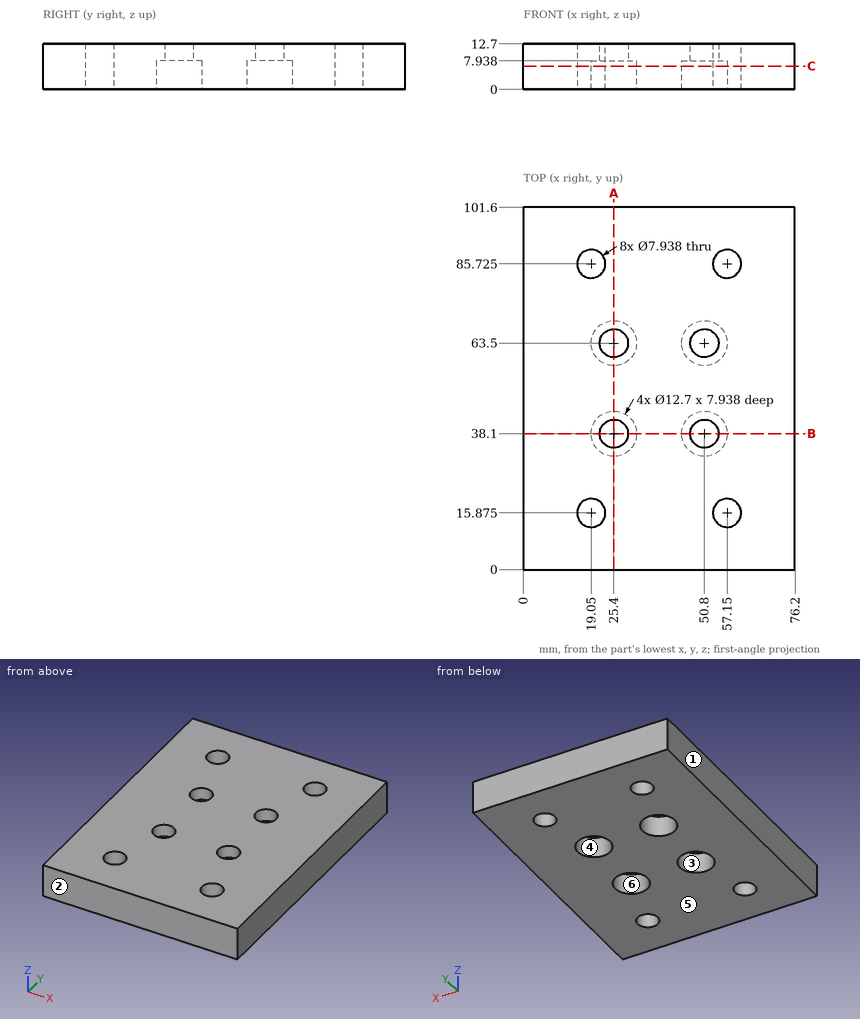
Part print with two shaded views. Sizes in mm from the minimum x, y, z corner. A direction names the side the tool comes from. Give positions to 0.01 mm unless a question says otherwise; leave off trailing zeros. Order: outer loops, then holes, each group sorted by start corner. A loop starts at its lowest first (then second) coordinate and runs counter-clockwise, first axis right, second up. Notation, with made-up numbers: M -37,-27.75 L -25,-27.75 A25 cw -25,-6.75 Z; hole C 8,9.5 d3. An arc over 180 degrees is marked long. Put each result on its own line as item: value.
Item 1: Drop a flat-ended pin along its axis: pin 1 Ø12.5 at (x, y) = (50.8, 63.5) entering from -Z. Give the stop position or say it passes through.
Results are:
pin 1: z = 7.94
Item 2: Cut at A-A on x = 25.4. Write the cut outline in (y, z).
Results are:
outline: M 0,0 L 31.75,0 L 31.75,7.94 L 34.13,7.94 L 34.13,12.7 L 0,12.7 Z; M 42.07,7.94 L 44.45,7.94 L 44.45,0 L 57.15,0 L 57.15,7.94 L 59.53,7.94 L 59.53,12.7 L 42.07,12.7 Z; M 67.47,7.94 L 69.85,7.94 L 69.85,0 L 101.6,0 L 101.6,12.7 L 67.47,12.7 Z
Item 3: Wall check: probe 1 along Y at (x, z) = (50.8, 9.3); probe 2 along X at (y, z) = (83, 2.5) (1 decimal); probe 3 along Y at (x, z) = (58.5, 5). Give the ranges that are in metal, low to high.
Results are:
probe 1: 0 to 34.13, 42.07 to 59.53, 67.47 to 101.6
probe 2: 0 to 16.2, 21.9 to 54.3, 60 to 76.2
probe 3: 0 to 12.14, 19.61 to 81.99, 89.46 to 101.6
Item 4: Cut at B-B on y = 38.1. Write the cut outline in (x, z).
Results are:
outline: M 0,0 L 19.05,0 L 19.05,7.94 L 21.43,7.94 L 21.43,12.7 L 0,12.7 Z; M 29.37,7.94 L 31.75,7.94 L 31.75,0 L 44.45,0 L 44.45,7.94 L 46.83,7.94 L 46.83,12.7 L 29.37,12.7 Z; M 54.77,7.94 L 57.15,7.94 L 57.15,0 L 76.2,0 L 76.2,12.7 L 54.77,12.7 Z
Item 5: Pull direction Y, two halves, no side cores. Call the marked faces 1, 2, 3 and 4: +Y half, -Y half, draft (parallel to the pull), parting line (faces both ways), or undercut.
Results are:
face 1: draft
face 2: -Y half
face 3: undercut
face 4: undercut
Item 6: Cut at C-C on z = 6.5. Count the separate pieces of the cut face and the enclosed holes in it, then the cut area to 3 significant figures.
Results are:
separate pieces: 1
enclosed holes: 8
area: 7,040 mm2
Item 7: Which spindle directions (+Z, -Z, +X, -X, +Y, -Y) get a long thin tool onto all of the face, cutting with end or side? Do the marked faces 5 and 6. Say none if no direction does.
Results are:
face 5: -Z, +X, -X, +Y, -Y
face 6: -Z
